Design review of the part built by this model. Coordinates are the model's own, in mm. A direction names the side the tool comes from. Round coordinates to 2 decimals unless told otherwise and drop trailing zeros. Write each loop counter-clockwise with the first axis right and the second up, starting at its lowest first coordinate (ties: lowest second). Pieces come first, ordered by that corner, then holes. Notation, with made-up numbers: M 33,64 L 42,64 A20 cw 42,76 Z; hole C -32.5,60.5 d5. An arc over 180 degrees is marked long. Use CSV: the item, a comma, the result in double quotes.
from build123d import *

# Parameters (mm, degrees)
CYLINDER003_R             = 1
CYLINDER003_DEPTH         = 5
CYLINDER001_R             = 1
CYLINDER001_DEPTH         = 5
CYLINDER002_R             = 1
CYLINDER002_DEPTH         = 5
BOX_W                     = 12
BOX_H                     = 6
BOX_DEPTH                 = 2
CYLINDER009_R             = 1.65
CYLINDER009_DEPTH         = 8
CHAMFER_SIZE              = 1.65
CYLINDER010_R             = 1.65
CYLINDER010_DEPTH         = 8
CHAMFER001_SIZE           = 1.65
CYLINDER_R                = 1
CYLINDER_DEPTH            = 5
BOX003_W                  = 34
BOX003_H                  = 34
BOX003_DEPTH              = 8
BOX002_W                  = 39
BOX002_H                  = 39
BOX002_DEPTH              = 4
CYLINDER004_R             = 29.9
CYLINDER004_DEPTH         = 10
CYLINDER006_R             = 4
CYLINDER006_DEPTH         = 6
FILLET004_R               = 4
CYLINDER008_R             = 4
CYLINDER008_DEPTH         = 6
FILLET005_R               = 4
BOX004_W                  = 5.5
BOX004_H                  = 5.5
BOX004_DEPTH              = 4
FILLET002_R               = 3
FILLET002_PLACEMENT_ANGLE = 180
FILLET001_R               = 3
FILLET001_PLACEMENT_ANGLE = 90
FILLET_R                  = 3
FILLET003_R               = 3
FILLET003_PLACEMENT_ANGLE = 90


with BuildPart() as cylinder003:
    # Cylinder003 → Cylinder003 (new body)
    with BuildSketch(Plane(origin=(14, -14, 1), x_dir=(1, 0, 0), z_dir=(0, 0, 1))):
        Circle(CYLINDER003_R)
    extrude(amount=CYLINDER003_DEPTH)


with BuildPart() as cylinder001:
    # Cylinder001 → Cylinder001 (new body)
    with BuildSketch(Plane(origin=(-14, 14, 1), x_dir=(1, 0, 0), z_dir=(0, 0, 1))):
        Circle(CYLINDER001_R)
    extrude(amount=CYLINDER001_DEPTH)


with BuildPart() as cylinder002:
    # Cylinder002 → Cylinder002 (new body)
    with BuildSketch(Plane(origin=(-14, -14, 1), x_dir=(1, 0, 0), z_dir=(0, 0, 1))):
        Circle(CYLINDER002_R)
    extrude(amount=CYLINDER002_DEPTH)


with BuildPart() as obj1:
    # Box → Box (new body)
    with BuildSketch(Plane(origin=(-6, 10.5, 0), x_dir=(1, 0, 0), z_dir=(0, 0, 1))):
        with Locations((6, 3)):
            Rectangle(BOX_W, BOX_H)
    extrude(amount=BOX_DEPTH)


with BuildPart() as chamfer001:
    # Cylinder009 → Cylinder009 (new body)
    with BuildSketch(Plane(origin=(0, -25, 0), x_dir=(1, 0, 0), z_dir=(0, 0, 1))):
        Circle(CYLINDER009_R)
    extrude(amount=CYLINDER009_DEPTH)

    # Chamfer
    chamfer_edges = [chamfer001.edges().sort_by_distance(p)[0] for p in [
        (-1.65, -25, 8),
    ]]
    chamfer(chamfer_edges, length=CHAMFER_SIZE)


with BuildPart() as chamfer002:
    # Cylinder010 → Cylinder010 (new body)
    with BuildSketch(Plane(origin=(0, 25, 0), x_dir=(1, 0, 0), z_dir=(0, 0, 1))):
        Circle(CYLINDER010_R)
    extrude(amount=CYLINDER010_DEPTH)

    # Chamfer001
    chamfer001_edges = [chamfer002.edges().sort_by_distance(p)[0] for p in [
        (-1.65, 25, 8),
    ]]
    chamfer(chamfer001_edges, length=CHAMFER001_SIZE)


with BuildPart() as obj2:
    # Cylinder → Cylinder (new body)
    with BuildSketch(Plane(origin=(14, 14, 1), x_dir=(1, 0, 0), z_dir=(0, 0, 1))):
        Circle(CYLINDER_R)
    extrude(amount=CYLINDER_DEPTH)

    # Fusion: union Cylinder003, Cylinder001, Cylinder002, obj1, Chamfer001, Chamfer002
    add(cylinder003.part)
    add(cylinder001.part)
    add(cylinder002.part)
    add(obj1.part)
    add(chamfer001.part)
    add(chamfer002.part)


with BuildPart() as rahmen_innen:
    # Box003 → Box003 (new body)
    with BuildSketch(Plane(origin=(-17, -17, 2), x_dir=(1, 0, 0), z_dir=(0, 0, 1))):
        with Locations((17, 17)):
            Rectangle(BOX003_W, BOX003_H)
    extrude(amount=BOX003_DEPTH)


with BuildPart() as rahmen_aussen:
    # Box002 → Box002 (new body)
    with BuildSketch(Plane(origin=(-19.5, -19.5, 6), x_dir=(1, 0, 0), z_dir=(0, 0, 1))):
        with Locations((19.5, 19.5)):
            Rectangle(BOX002_W, BOX002_H)
    extrude(amount=BOX002_DEPTH)


with BuildPart() as cut001:
    # Cylinder004 → Cylinder004 (new body)
    with BuildSketch(Plane.XY):
        Circle(CYLINDER004_R)
    extrude(amount=CYLINDER004_DEPTH)

    # Cut: cut Rahmen_Aussen
    add(rahmen_aussen.part, mode=Mode.SUBTRACT)

    # Cut001: cut Rahmen_Innen
    add(rahmen_innen.part, mode=Mode.SUBTRACT)


with BuildPart() as fillet004:
    # Cylinder006 → Cylinder006 (new body)
    with BuildSketch(Plane(origin=(-25, 0, 10), x_dir=(1, 0, 0), z_dir=(0, 0, 1))):
        Circle(CYLINDER006_R)
    extrude(amount=CYLINDER006_DEPTH)

    # Fillet004
    fillet004_edges = [fillet004.edges().sort_by_distance(p)[0] for p in [
        (-29, 0, 16),
    ]]
    fillet(fillet004_edges, radius=FILLET004_R)


with BuildPart() as fillet005:
    # Cylinder008 → Cylinder008 (new body)
    with BuildSketch(Plane(origin=(25, 0, 10), x_dir=(1, 0, 0), z_dir=(0, 0, 1))):
        Circle(CYLINDER008_R)
    extrude(amount=CYLINDER008_DEPTH)

    # Fillet005
    fillet005_edges = [fillet005.edges().sort_by_distance(p)[0] for p in [
        (21, 0, 16),
    ]]
    fillet(fillet005_edges, radius=FILLET005_R)


with BuildPart() as obj3:
    # Box004 → Box004 (new body)
    with BuildSketch(Plane(origin=(11.5, 11.5, 2), x_dir=(1, 0, 0), z_dir=(0, 0, 1))):
        with Locations((2.75, 2.75)):
            Rectangle(BOX004_W, BOX004_H)
    extrude(amount=BOX004_DEPTH)


with BuildPart() as fillet002:
    # Fillet002 base: copy of obj3
    add(obj3.part)

    # Fillet002
    fillet002_edges = [fillet002.edges().sort_by_distance(p)[0] for p in [
        (11.5, 11.5, 4),
    ]]
    fillet(fillet002_edges, radius=FILLET002_R)


with BuildPart() as fillet002_1:
    # Fillet002 placement: moved
    add(fillet002.part.rotate(Axis((0, 0, 0), (0, 0, 1)), FILLET002_PLACEMENT_ANGLE))


with BuildPart() as fillet001:
    # Fillet001 base: copy of obj3
    add(obj3.part)

    # Fillet001
    fillet001_edges = [fillet001.edges().sort_by_distance(p)[0] for p in [
        (11.5, 11.5, 4),
    ]]
    fillet(fillet001_edges, radius=FILLET001_R)


with BuildPart() as fillet001_1:
    # Fillet001 placement: moved
    add(fillet001.part.rotate(Axis((0, 0, 0), (0, 0, 1)), FILLET001_PLACEMENT_ANGLE))


with BuildPart() as fillet_body:
    # Fillet base: copy of obj3
    add(obj3.part)

    # Fillet
    fillet_edges = [fillet_body.edges().sort_by_distance(p)[0] for p in [
        (11.5, 11.5, 4),
    ]]
    fillet(fillet_edges, radius=FILLET_R)


with BuildPart() as cut002:
    # Fillet003 base: copy of obj3
    add(obj3.part)

    # Fillet003
    fillet003_edges = [cut002.edges().sort_by_distance(p)[0] for p in [
        (11.5, 11.5, 4),
    ]]
    fillet(fillet003_edges, radius=FILLET003_R)


with BuildPart() as cut002_1:
    # Fillet003 placement: moved
    add(cut002.part.rotate(Axis((0, 0, 0), (0, 0, -1)), FILLET003_PLACEMENT_ANGLE))

    # Fusion001: union Fillet002, Fillet001, Fillet body
    add(fillet002_1.part)
    add(fillet001_1.part)
    add(fillet_body.part)

    # Fusion002: union Cut001, Fillet004, Fillet005
    add(cut001.part)
    add(fillet004.part)
    add(fillet005.part)

    # Cut002: cut obj2
    add(obj2.part, mode=Mode.SUBTRACT)


solid = cut002_1.part
1) Add section C-C on x = 25. Write out the cut boundary in (y, z), then the cut area to 3 significant figures.
Answers:
outline,"M -16.4,0 L 16.4,0 L 16.4,10 L 4,10 L 4,12 A4 ccw -4,12 L -4,10 L -16.4,10 Z"
area,"369 mm²"
2) Add section B-B on y = 0. Write out the cut boundary in (x, z).
Answers:
outline,"M -29.9,0 L 29.9,0 L 29.9,10 L 29,10 L 29,12 A4 ccw 21,12 L 21,10 L 19.5,10 L 19.5,6 L 17,6 L 17,2 L -17,2 L -17,6 L -19.5,6 L -19.5,10 L -21,10 L -21,12 A4 ccw -29,12 L -29,10 L -29.9,10 Z"
3) Add section A-A on z = 3.25. Write out the cut boundary in (x, y).
Answers:
outline,"C 0,0 d59.8; hole M -17,-11.5 L -14.5,-11.5 A3 cw -11.5,-14.5 L -11.5,-17 L 11.5,-17 L 11.5,-14.5 A3 cw 14.5,-11.5 L 17,-11.5 L 17,11.5 L 14.5,11.5 A3 cw 11.5,14.5 L 11.5,17 L -11.5,17 L -11.5,14.5 A3 cw -14.5,11.5 L -17,11.5 Z; hole C -14,-14 d2; hole C -14,14 d2; hole C 0,-25 d3.3; hole C 0,25 d3.3; hole C 14,-14 d2; hole C 14,14 d2"
4) For pin 1 Ø3 at (x, z) = (15, 4.5) entering from -Y; pin 2 Ø3 at (y, z) = (-16.5, 4.5) entering from -X; pin 3 Ø0.6 at (x, y) = (-14, 14) entering from +Z; pin 4 Ø5 at (y, z) = (19, 13.5) entering from +X, all flat-tipped, find the tip position at first contact; note any pin that passes through.
Answers:
pin 1,"y = -26.68"
pin 2,"x = -25.87"
pin 3,"z = 1"
pin 4,"through"
5) The part is to be moulded in two halves that separate along X. For faces 4 (the face through (13.797, -26.526, 4.93)), 5 (the face through (-12.4, 12.36, 4.03)), 6 (the face through (19.5, 0, 8)), 7 (the face through (0, 0, 0)), say which applies: released by +X, released by -X, zero draft, split by the parting line, or undercut.
Answers:
face 4,"split by the parting line"
face 5,"undercut"
face 6,"undercut"
face 7,"zero draft"
6) Wall thickness on line 1 along Y through (x, z) = (0, 5); line 2 along Y through (x, z) = (14, 4.6); line 3 along X through (y, z) = (1, 4): over which ranges is each line inside the solid? List them lowest first. Write a range as [from, to].
Answers:
line 1,"[-29.9, -26.65], [-23.35, -17], [17, 23.35], [26.65, 29.9]"
line 2,"[-26.42, -15], [-13, -11.54], [11.54, 13], [15, 26.42]"
line 3,"[-29.88, -17], [17, 29.88]"
7) Add section D-D on y = 6.5. Write out the cut boundary in (x, z).
Answers:
outline,"M -29.18,0 L 29.18,0 L 29.18,10 L 19.5,10 L 19.5,6 L 17,6 L 17,2 L -17,2 L -17,6 L -19.5,6 L -19.5,10 L -29.18,10 Z"
8) Machinability: for faces 1 (the face through (0, 10.5, 1)), 2 (the face through (16, -11.5, 4)), 3 (the face through (-0.215, 26.636, 3.131)), which of the approach directions +Z, -Z, +X, -X, +Y, -Y give a long, thin tool a straight path to every point of the face, cutting with its end or side? Answer none if there is none.
Answers:
face 1,"+Z, -Z"
face 2,"+Z"
face 3,"-Z"
